from build123d import *

# Parameters (mm, degrees)
SKETCH1_R                 = 6.477
SKETCH1_R_2               = 2.19075
SKETCH1_R_3               = 8.89
BOSS_EXTRUDE1_DEPTH       = 9.525
F_1_0MM_DOWEL_HOLE1_D     = 3.0226
F_1_0MM_DOWEL_HOLE1_DEPTH = 9.99998
F_1_0MM_DOWEL_HOLE1_TIP   = 0.908080654


with BuildPart() as part:
    # Sketch1 → Boss-Extrude1 (new body)
    with BuildSketch(Plane.XZ):
        with BuildLine():
            Line((-35.56, -19.05), (35.56, -19.05))
            ThreePointArc((35.56, -19.05), (37.356051224, -18.306051224), (38.1, -16.51))
            Line((38.1, -16.51), (38.1, 16.51))
            ThreePointArc((38.1, 16.51), (37.356051224, 18.306051224), (35.56, 19.05))
            Line((35.56, 19.05), (-35.56, 19.05))
            ThreePointArc((-35.56, 19.05), (-37.356051224, 18.306051224), (-38.1, 16.51))
            Line((-38.1, 16.51), (-38.1, -16.51))
            ThreePointArc((-38.1, -16.51), (-37.356051224, -18.306051224), (-35.56, -19.05))
        make_face()
        with Locations(Location((-21.59, 0, 0), (0, 0, 270))):
            Circle(SKETCH1_R, mode=Mode.SUBTRACT)
        with Locations(Location((-21.59, -10.31875, 0), (0, 0, 270))):
            Circle(SKETCH1_R_2, mode=Mode.SUBTRACT)
        with Locations(Location((-21.59, 10.31875, 0), (0, 0, 270))):
            Circle(SKETCH1_R_2, mode=Mode.SUBTRACT)
        with Locations(Location((21.59, 0, 0), (0, 0, 270))):
            Circle(SKETCH1_R_3, mode=Mode.SUBTRACT)
    extrude(amount=-BOSS_EXTRUDE1_DEPTH)

    # Ø1.0mm Dowel Hole1
    with Locations(Plane(origin=(0, 9.525, 0), x_dir=(1, 0, 0), z_dir=(0, 1, 0))):
        with Locations((-34.29, 15.24), (-34.29, -15.24), (34.29, -15.24), (34.29, 15.24)):
            Hole(F_1_0MM_DOWEL_HOLE1_D / 2, depth=F_1_0MM_DOWEL_HOLE1_DEPTH)
            with Locations((0, 0, -(F_1_0MM_DOWEL_HOLE1_DEPTH + F_1_0MM_DOWEL_HOLE1_TIP / 2))):  # 118° drill point
                Cone(0, F_1_0MM_DOWEL_HOLE1_D / 2, F_1_0MM_DOWEL_HOLE1_TIP, mode=Mode.SUBTRACT)


solid = part.part
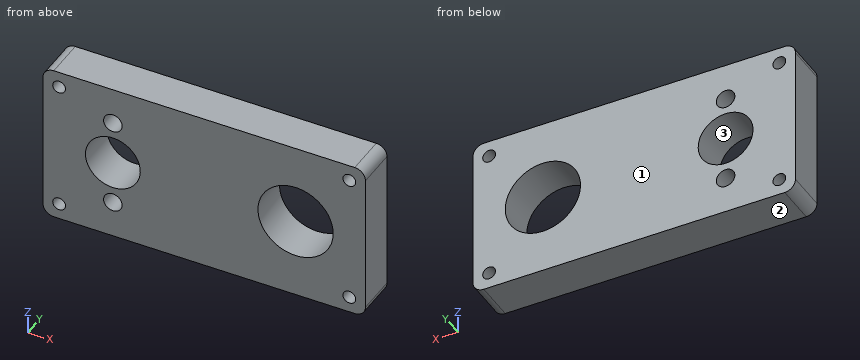
Source: CAD feature listing. Evaluate the final solid. Frame: model axes, mm. Face numbers are marked on the shaded views. Round coordinates to 2 decimals unless told otherwise and drop trailing zeros. Loops run counter-clockwise (first coordinate to the right, second up) from the corner with the lowest first, then second, coordinate; pieces in that order, holes last. Notation, with made-up numbers: (78, 21) -> (134, 21) arc R19 cw to (134, 37) -> close; hole circle Ø8 at (67, 7). An arc over 180 degrees is marked (long way). Answer as a JSON object with one key per item and string values. Group by question number.
Q1. Mould query, pull axis Z, two halves, no side actions, for the marked faces 1, 2 and 3. Classes: pulls with the +Z half, pulls with the -Z half, needs draft (parallel to the pull), parting line crosses it, or undercut.
Q2. Section query B-B (y = 4.5). State how many separate pieces and enclosed holes the cut face has, plus the area to 3 significant figures.
Q3. Ray query, line 1 (Z direction, x = 34.29, y = 4.25); line 2 (X direction, y = 5.5, z = 15.24); line 3 (X direction, y = 2.75, z = -4.5). Return the intervals inside material, ascending. Write a range as from..to.
Q4. Section query A-A (z = 15.24). Output: boundary loops of the cut face in (x, y) (3 decimals), plus the area to 3 significant figures.
Q5. Section query D-D (x = -34.29). Output: boundary loops of the cut face in (y, z) (3 decimals).
Completed:
{
 "1": {"face 1": "needs draft", "face 2": "pulls with the -Z half", "face 3": "undercut"},
 "2": {"separate pieces": "1", "enclosed holes": "8", "area": "2,460 mm²"},
 "3": {"line 1": "-19.05..-16.75, -13.73..13.73, 16.75..19.05", "line 2": "-38.1..-35.8, -32.78..32.78, 35.8..38.1", "line 3": "-38.1..-26.25, -16.93..13.92, 29.26..38.1"},
 "4": {"outline": "(-38.1, 0) -> (-35.801, 0) -> (-35.801, 9.525) -> (-38.1, 9.525) -> close; (-32.779, 0) -> (32.779, 0) -> (32.779, 9.525) -> (-32.779, 9.525) -> close; (35.801, 0) -> (38.1, 0) -> (38.1, 9.525) -> (35.801, 9.525) -> close", "area": "668 mm²"},
 "5": {"outline": "(0, -19.05) -> (9.525, -19.05) -> (9.525, -16.751) -> (0, -16.751) -> close; (0, -13.729) -> (9.525, -13.729) -> (9.525, 13.729) -> (0, 13.729) -> close; (0, 16.751) -> (9.525, 16.751) -> (9.525, 19.05) -> (0, 19.05) -> close"}
}
